from build123d import *

# Parameters (mm, degrees)
F0_W        = 46
F0_H        = 200
F0_W_2      = 43
F0_H_2      = 53
F0_R        = 13
F1_DEPTH    = 11.8
F0_R_2      = 14
F1_FACE_W   = 46
F1_FACE_H   = 200
F1_FACE_W_2 = 43
F1_FACE_H_2 = 53
F1_FACE_R   = 13
F2_DEPTH    = 0.5
F3_W        = 7
F3_H        = 93.5
F4_DEPTH    = 5
F0_R_3      = 11.5
F5_DEPTH    = 1


with BuildPart() as f1:
    # F0 (on Top) → F1 (new body)
    with BuildSketch(Plane.XY):
        with Locations((0.973917, 4.583021)):
            Rectangle(F0_W, F0_H)
        with Locations((0.973917, 24.583021)):
            Rectangle(F0_W_2, F0_H_2, mode=Mode.SUBTRACT)
        with Locations((0.973917, 74.583021)):
            Circle(F0_R, mode=Mode.SUBTRACT)
    extrude(amount=F1_DEPTH)

    # F0 (on Top) + F1_face (on face) → F2 (join)
    with BuildSketch(Plane.XY):
        with Locations((0.973917, 24.583021)):
            Rectangle(F0_W_2, F0_H_2)
        with Locations((0.973917, 24.583021)):
            Circle(F0_R_2, mode=Mode.SUBTRACT)
    with BuildSketch(Plane(origin=(0.973917, -8.365981, 11.8), x_dir=(1, 0, 0), z_dir=(0, 0, 1))):
        with Locations((0, 12.949002)):
            Rectangle(F1_FACE_W, F1_FACE_H)
        with Locations((0, 32.949002)):
            Rectangle(F1_FACE_W_2, F1_FACE_H_2, mode=Mode.SUBTRACT)
        with Locations((0, 82.949002)):
            Circle(F1_FACE_R, mode=Mode.SUBTRACT)
    extrude(amount=F2_DEPTH)

    # F3 (on face) → F4 (cut)
    with BuildSketch(Plane.XY.offset(12.3)):
        with Locations((0.973917, -48.666979)):
            Rectangle(F3_W, F3_H)
    extrude(amount=-F4_DEPTH, mode=Mode.SUBTRACT)

    # F0 (on Top) → F5 (join)
    with BuildSketch(Plane.XY):
        with Locations((0.973917, 74.583021)):
            Circle(F0_R)
        with Locations((0.973917, 74.583021)):
            Circle(F0_R_3, mode=Mode.SUBTRACT)
    extrude(amount=F5_DEPTH)


solid = f1.part
Work out the finished part from the listing and answer in its coordinate system (mm). A direction names the side the tool comes from. Round coordinates to 2 decimals unless told otherwise and drop trailing zeros. Write each loop counter-clockwise with the first axis right and the second up, starting at its lowest first coordinate (ties: lowest second). Pieces come first, ordered by that corner, then holes.
1) A cutting plane is placed at A-A (y = 35.5). Give the vertices of the cut face in (x, z).
2) A tool of negligible diameter and unlimited length cuts with its end or side. For faces 1 (the flat face through (1, 6, 0)), 2 (the flat face through (1, -48, 7.3)), 3 (the flat face through (-14, 25, 0.5)), from which of +Z, -Z, +X, -X, +Y, -Y can it reach the whole face along a straight path? Write none if from no direction.
3) Given pin 1 Ø5.5 at (x, y) = (-0.5, -42) entering from +Z; pin 2 Ø8 at (x, y) = (15.5, 12.5) entering from +Z, each flat-ended and moving along its own axis, determine where each tip first touches the part or whether it passes through.
4) Straight lines are drawn through the part: line 1 (Y direction, x = 7, z = 8); line 2 (X direction, y = -40, z = 10.75); line 3 (X direction, y = 19, z = 8.5). For each, find the intervals that lie inside material, in ascending order.
5) A cutting plane is placed at C-C (y = -71). Give the vertices of the cut face in (x, z).
6) A cutting plane is placed at D-D (x = -0.5). Give the vertices of the cut face in (y, z).
7) A cutting plane is placed at B-B (z = 10.5). Give the vertices of the cut face in (x, y), plus the area to 3 significant figures.
8) The mould has two halves that part along X. Classify faces 4 (the cylindrical face through (6.28, 64.38, 0.49)), 5 (the flat face through (-4, -16, 12.3)), 6 (the flat face through (23.974, 3, 6)), 7 (the cylindrical face through (-1.84, 61.89, 6.57)): pulls with the +X half, pulls with the -X half, needs draft (parallel to the pull), parting line crosses it, or undercut.
Completed:
1. outline: (-22.03, 0) - (-7.79, 0) - (-7.79, 0.5) - (-20.53, 0.5) - (-20.53, 12.3) - (-22.03, 12.3) - close; (9.74, 0) - (23.97, 0) - (23.97, 12.3) - (22.47, 12.3) - (22.47, 0.5) - (9.74, 0.5) - close
2. face 1: -Z, +X, -X, +Y, -Y
2. face 2: +Z, -Y
2. face 3: +Z
3. pin 1: stops at z = 12.3
3. pin 2: stops at z = 0.5
4. line 1: y = -95.42 to -1.92, 51.08 to 63.06, 86.1 to 104.58
4. line 2: x = -22.03 to -2.53, 4.47 to 23.97
4. line 3: x = -22.03 to -20.53, 22.47 to 23.97
5. outline: (-22.03, 0) - (23.97, 0) - (23.97, 12.3) - (4.47, 12.3) - (4.47, 7.3) - (-2.53, 7.3) - (-2.53, 12.3) - (-22.03, 12.3) - close
6. outline: (-95.42, 0) - (10.66, 0) - (10.66, 0.5) - (-1.92, 0.5) - (-1.92, 7.3) - (-95.42, 7.3) - close; (38.51, 0) - (63.18, 0) - (63.18, 1) - (61.67, 1) - (61.67, 12.3) - (51.08, 12.3) - (51.08, 0.5) - (38.51, 0.5) - close; (85.99, 0) - (104.58, 0) - (104.58, 12.3) - (87.5, 12.3) - (87.5, 1) - (85.99, 1) - close
7. outline: (-22.03, -95.42) - (-2.53, -95.42) - (-2.53, -1.92) - (-20.53, -1.92) - (-20.53, 51.08) - (22.47, 51.08) - (22.47, -1.92) - (4.47, -1.92) - (4.47, -95.42) - (23.97, -95.42) - (23.97, 104.58) - (-22.03, 104.58) - close; hole circle Ø26 at (0.97, 74.58)
7. area: 5,740 mm2
8. face 4: undercut
8. face 5: needs draft
8. face 6: pulls with the +X half
8. face 7: undercut
